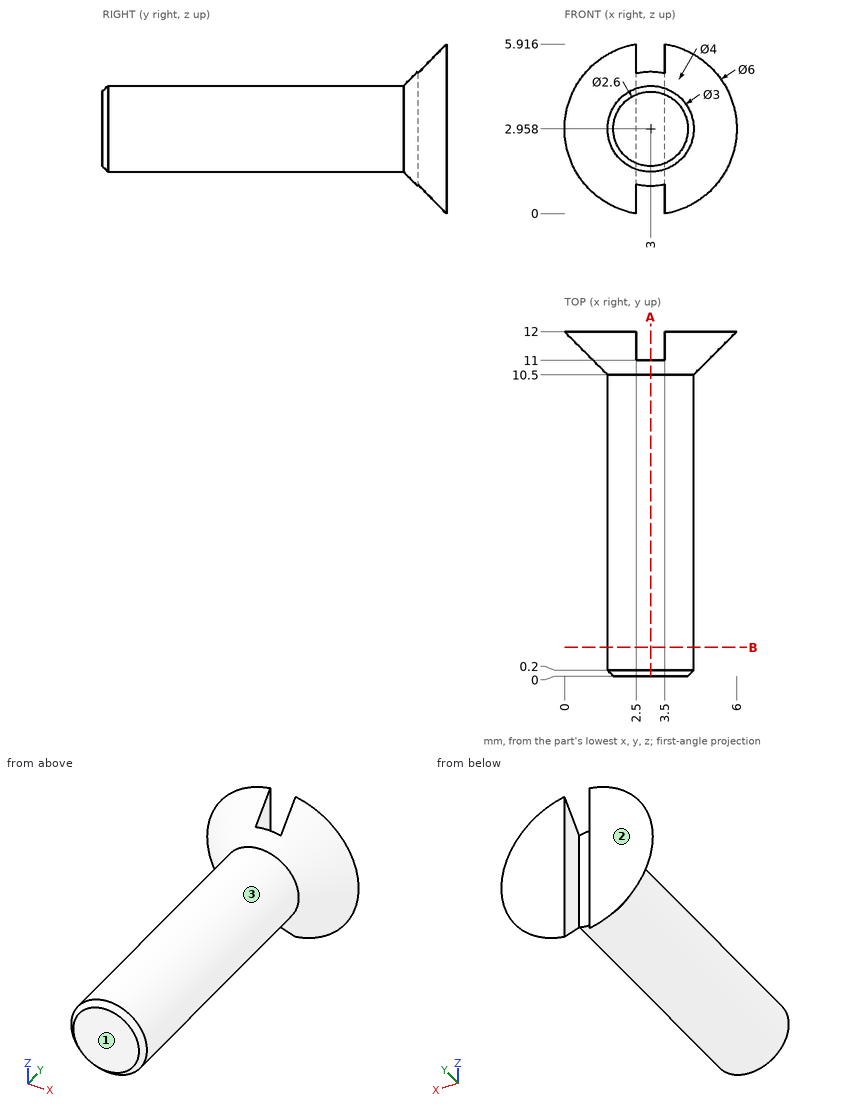
Geometry check sheet. Reference: drawing and pictorial views, mm from the part's lowest x, y, z. Round coordinates to 2 decimals unless told otherwise and drop trailing zeros. Order: outer loops, then holes, each group sorted by start corner. A loop starts at its lowest first (then second) coordinate and runs counter-clockwise, first axis right, second up. Notation, with made-up numbers: (9.25, 20.5) - (24.25, 20.5) arc R13 cw to (24.25, 42.5) - close; hole circle Ø9 at (18, 30.5). An arc over 180 degrees is marked (long way). Use a Markdown table: item, result. Add a question column.
1) Gauge pin test, flat ends, axial feed: P1, Ø2, axis at x = 4.5, y = 3, coming from the +Z side; P2, Ø1.1, axis at x = 3, z = 3.5, coming from the +Y side; P3, Ø1.5, axis at y = 5, z = 5, coming from the -X side; P4, Ø3, axis at y = 6.5, z = 0.5, coming from the -X side. Record the tip position at first contact, or that the pin passes through.
2) Section check A-A (x = 3). Record the cut outline in (y, z), then the cut area to 3 significant figures.
3) Thickness scan on line 1 along Y through (x, z) = (3.2, 3.15); line 2 along Z through (x, y) = (3.45, 6); line 3 along X through (y, z) = (6.5, 1.9). Record the ranges inside material, lowest first.
4) Mould release check, pull along Y, two halves, no side actions. Record for the marked faces 1, 2 and 3: released by +Y, released by -Y, zero draft, split by the parting line, or undercut.
5) Section check B-B (y = 1). Record the cut outline in (x, z), then the cut area to 3 significant figures.
Established:
| question | item | result |
|---|---|---|
| 1 | P1 | z = 4.37 |
| 1 | P2 | y = 12 |
| 1 | P3 | x = 2.24 |
| 1 | P4 | x = 1.85 |
| 2 | outline | (0, 1.66) - (0.2, 1.46) - (10.5, 1.46) - (11, 0.96) - (11, 4.96) - (10.5, 4.46) - (0.2, 4.46) - (0, 4.26) - close |
| 2 | area | 33.2 mm2 |
| 3 | line 1 | 0 to 11 |
| 3 | line 2 | 1.53 to 4.39 |
| 3 | line 3 | 1.94 to 4.06 |
| 4 | face 1 | released by -Y |
| 4 | face 2 | released by +Y |
| 4 | face 3 | zero draft |
| 5 | outline | circle Ø3 at (3, 2.96) |
| 5 | area | 7.07 mm2 |
